Here's how the part is built. I have some questions about the finished solid (model axes, mm). A direction names the side the tool comes from. Coordinates: 2 decimals unless noted, no trailing zeros. Order: outer loops, then holes, each group sorted by start corner. A loop starts at its lowest first (then second) coordinate and runs counter-clockwise, first axis right, second up. Notation, with made-up numbers: (8.5, 3.25) - (38.5, 3.25) arc R23 cw to (38.5, 18.25) - close; hole circle Ø10 at (-12.75, 10.25). An arc over 180 degrees is marked (long way). Answer in a Markdown table with one row per item. Add a question column.
Item 1: Thinking about a two-plate mould opening in X: for faces 1 (the flat face through (2, 4.5, 1)), 2 (the flat face through (-3.253, 0.986, -11.798)), 3 (the cylindrical face through (-0.25, 3.23, -1.89)), which applies, +X half, -X half, draft (parallel to the pull), parting line (faces both ways), or undercut?
Item 2: I want a section at C-C (y = 4.05). Please give me the cut outline in (x, z), plus the area to 3 significant figures.
Item 3: I want a section at A-A (x = 0). Please give me the cut outline in (y, z), plus the area to 3 significant figures.
Item 4: If I drill on line 1 along X through (y, z) = (3.55, 0); line 2 along Z through (x, y) = (-1.5, 3.55), over which ranges is the centre line in solid material (lowest first)? Write a range as from..to.
Item 5: I want a section at D-D (y = 1.5). Please give me the cut outline in (x, z).
Item 6: Will these pins go through, and if not, where does the flat tip stop? pin 1 Ø4 at (x, z) = (0.5, 0.5) entering from +Y; pin 2 Ø2.5 at (x, z) = (0, 0) entering from +Y.
Item 7: I want a section at B-B (z = 0). Please give me the cut outline in (x, y), plus the area to 3 significant figures.
Item 8: On a 3-axis mill with a long thin cutter (end or side, diameter ignored), from which of +Z, -Z, +X, -X, +Y, -Y can I reach the whole of each face in a straight line? I mean faces 4 (the flat face through (0, 2, 0)), 5 (the flat face through (0, 0, -11)). Say none if no direction works.
```python
from build123d import *

# Parameters (mm, degrees)
BOSS_EXTRUDE1_DEPTH = 2
SKETCH2_R           = 4
SKETCH2_R_2         = 1.906385326
BOSS_EXTRUDE2_DEPTH = 2.5


with BuildPart() as part:
    # Sketch1 → Boss-Extrude1 (new body)
    with BuildSketch(Plane(origin=(0, 0, 0), x_dir=(1, 0, 0), z_dir=(0, 1, 0))):
        with BuildLine():
            Line((3.991833672, 0.255468066), (2.534814382, 23.022222222))
            ThreePointArc((2.534814382, 23.022222222), (0, 25.4), (-2.534814382, 23.022222222))
            Line((-2.534814382, 23.022222222), (-3.991833672, 0.255468066))
            ThreePointArc((-3.991833672, 0.255468066), (0, -4), (3.991833672, 0.255468066))
        make_face()
    extrude(amount=BOSS_EXTRUDE1_DEPTH)

    # Sketch2 → Boss-Extrude2 (add)
    with BuildSketch(Plane(origin=(0, 2, 0), x_dir=(1, 0, 0), z_dir=(0, 1, 0))):
        Circle(SKETCH2_R)
        Circle(SKETCH2_R_2, mode=Mode.SUBTRACT)
    extrude(amount=BOSS_EXTRUDE2_DEPTH)


solid = part.part
```
Values follow:
| question | item | result |
|---|---|---|
| 1 | face 1 | draft |
| 1 | face 2 | -X half |
| 1 | face 3 | undercut |
| 2 | outline | circle Ø8 at (0, 0); hole circle Ø3.81 at (0, 0) |
| 2 | area | 38.8 mm^2 |
| 3 | outline | (0, -25.4) - (2, -25.4) - (2, -4) - (4.5, -4) - (4.5, -1.91) - (2, -1.91) - (2, 1.91) - (4.5, 1.91) - (4.5, 4) - (0, 4) - close |
| 3 | area | 69.3 mm^2 |
| 4 | line 1 | x = -4..-1.91, 1.91..4 |
| 4 | line 2 | z = -3.71..-1.18, 1.18..3.71 |
| 5 | outline | (-3.99, -0.26) - (-2.53, -23.02) arc R2.54 ccw to (2.53, -23.02) - (3.99, -0.26) arc R4 ccw (long way) to start |
| 6 | pin 1 | stops at y = 4.5 |
| 6 | pin 2 | stops at y = 2 |
| 7 | outline | (-4, 0) - (4, 0) - (4, 4.5) - (1.91, 4.5) - (1.91, 2) - (-1.91, 2) - (-1.91, 4.5) - (-4, 4.5) - close |
| 7 | area | 26.5 mm^2 |
| 8 | face 4 | +Y |
| 8 | face 5 | +Z, -Z, +X, -X, -Y |
